from build123d import *

# Parameters (mm, degrees)
SKETCH3_W           = 20.4
SKETCH3_H           = 15.3
SKETCH3_R           = 0.5
SKETCH3_R_2         = 0.375
BOSS_EXTRUDE2_DEPTH = 0.825
SKETCH5_R           = 1
SKETCH5_R_2         = 0.5
SKETCH5_R_3         = 0.725
SKETCH5_R_4         = 0.375
BOSS_EXTRUDE3_DEPTH = 0.05


with BuildPart() as part:
    # Sketch3 → Boss-Extrude2 (new body, symmetric)
    with BuildSketch(Plane(origin=(0, 0, 0), x_dir=(1, 0, 0), z_dir=(0, 1, 0))):
        Rectangle(SKETCH3_W, SKETCH3_H)
        with Locations((-2.54, 5.11)):
            Circle(SKETCH3_R, mode=Mode.SUBTRACT)
        with Locations((0, 5.11)):
            Circle(SKETCH3_R, mode=Mode.SUBTRACT)
        with Locations((2.54, 5.11)):
            Circle(SKETCH3_R, mode=Mode.SUBTRACT)
        with Locations((-7.76, -2.57)):
            Circle(SKETCH3_R_2, mode=Mode.SUBTRACT)
        with Locations((-7.76, -5.11)):
            Circle(SKETCH3_R_2, mode=Mode.SUBTRACT)
        with Locations((7.76, -2.57)):
            Circle(SKETCH3_R_2, mode=Mode.SUBTRACT)
        with Locations((7.76, -5.11)):
            Circle(SKETCH3_R_2, mode=Mode.SUBTRACT)
        with Locations((6.260003, -3.84)):
            Circle(SKETCH3_R_2, mode=Mode.SUBTRACT)
        with Locations((-3.81, 1.3)):
            Circle(SKETCH3_R, mode=Mode.SUBTRACT)
        with Locations((3.81, 1.3)):
            Circle(SKETCH3_R, mode=Mode.SUBTRACT)
    extrude(amount=BOSS_EXTRUDE2_DEPTH, both=True)

    # Sketch5 → Boss-Extrude3 (add)
    with BuildSketch(Plane(origin=(0, 0.825, 0), x_dir=(1, 0, 0), z_dir=(0, 1, 0))):
        with Locations((-2.54, 5.11)):
            Circle(SKETCH5_R)
        with Locations((-2.54, 5.11)):
            Circle(SKETCH5_R_2, mode=Mode.SUBTRACT)
        with Locations((0, 5.11)):
            Circle(SKETCH5_R)
        with Locations((0, 5.11)):
            Circle(SKETCH5_R_2, mode=Mode.SUBTRACT)
        with Locations((2.54, 5.11)):
            Circle(SKETCH5_R)
        with Locations((2.54, 5.11)):
            Circle(SKETCH5_R_2, mode=Mode.SUBTRACT)
        with Locations((3.81, 1.3)):
            Circle(SKETCH5_R)
        with Locations((3.81, 1.3)):
            Circle(SKETCH5_R_2, mode=Mode.SUBTRACT)
        with Locations((-3.81, 1.3)):
            Circle(SKETCH5_R)
        with Locations((-3.81, 1.3)):
            Circle(SKETCH5_R_2, mode=Mode.SUBTRACT)
        with Locations((-7.76, -2.57)):
            Circle(SKETCH5_R_3)
        with Locations((-7.76, -2.57)):
            Circle(SKETCH5_R_4, mode=Mode.SUBTRACT)
        with Locations((-7.76, -5.11)):
            Circle(SKETCH5_R_3)
        with Locations((-7.76, -5.11)):
            Circle(SKETCH5_R_4, mode=Mode.SUBTRACT)
        with Locations((6.260003, -3.84)):
            Circle(SKETCH5_R_3)
        with Locations((6.260003, -3.84)):
            Circle(SKETCH5_R_4, mode=Mode.SUBTRACT)
        with Locations((7.76, -5.11)):
            Circle(SKETCH5_R_3)
        with Locations((7.76, -5.11)):
            Circle(SKETCH5_R_4, mode=Mode.SUBTRACT)
        with Locations((7.76, -2.57)):
            Circle(SKETCH5_R_3)
        with Locations((7.76, -2.57)):
            Circle(SKETCH5_R_4, mode=Mode.SUBTRACT)
    boss_extrude3 = extrude(amount=BOSS_EXTRUDE3_DEPTH)

    # Mirror1: Boss-Extrude3 across plane
    add(boss_extrude3.mirror(Plane.ZX))


solid = part.part
Geometry: final body of the model. Coordinates: model frame, mm. Give positions to 0.01 mm unless a question says otherwise; leave off trailing zeros. Loops run counter-clockwise (first coordinate to the right, second up) from the corner with the lowest first, then second, coordinate; pieces in that order, holes last. Notation, with made-up numbers: (63, -8.75) -> (117, -8.75) arc R20 ccw to (117, 16.25) -> close; hole circle Ø9 at (50.25, 7.5). An arc over 180 degrees is marked (long way). Put each result on its own line as item: value.
1. Cut plane C-C (y = -0.45). Count the separate pieces of the cut face and the enclosed holes in it, plus the area to 3 significant figures.
Taken from the geometry:
separate pieces: 1
enclosed holes: 10
area: 306 mm2
2. Pull-direction query (Z, two-part tool) for faces 1 (the flat face through (0, 0, 7.65)), 2 (the cylindrical face through (-3.04, 0.01, -5.13)), 3 (the flat face through (10.2, 0, 0)); classes: released by +Z, released by -Z, zero draft, split by the parting line, or undercut.
Taken from the geometry:
face 1: released by +Z
face 2: undercut
face 3: zero draft
3. Cut plane A-A (x = 2.54). Return the cut outline in (y, z) (3 decimals).
Taken from the geometry:
outline: (-0.875, -6.11) -> (-0.825, -6.11) -> (-0.825, -7.65) -> (0.825, -7.65) -> (0.825, -6.11) -> (0.875, -6.11) -> (0.875, -5.61) -> (-0.875, -5.61) -> close; (-0.875, -4.61) -> (0.875, -4.61) -> (0.875, -4.11) -> (0.825, -4.11) -> (0.825, 7.65) -> (-0.825, 7.65) -> (-0.825, -4.11) -> (-0.875, -4.11) -> close
4. Cut plane B-B (z = -1.3). Return the cut outline in (x, y) (3 decimals), plus the area to 3 significant figures.
Taken from the geometry:
outline: (-10.2, -0.825) -> (-4.81, -0.825) -> (-4.81, -0.875) -> (-4.31, -0.875) -> (-4.31, 0.875) -> (-4.81, 0.875) -> (-4.81, 0.825) -> (-10.2, 0.825) -> close; (-3.31, -0.875) -> (-2.81, -0.875) -> (-2.81, -0.825) -> (2.81, -0.825) -> (2.81, -0.875) -> (3.31, -0.875) -> (3.31, 0.875) -> (2.81, 0.875) -> (2.81, 0.825) -> (-2.81, 0.825) -> (-2.81, 0.875) -> (-3.31, 0.875) -> close; (4.31, -0.875) -> (4.81, -0.875) -> (4.81, -0.825) -> (10.2, -0.825) -> (10.2, 0.825) -> (4.81, 0.825) -> (4.81, 0.875) -> (4.31, 0.875) -> close
area: 30.6 mm2
5. Cut plane D-D (x = -7.76). Return the cut outline in (y, z) (3 decimals).
Taken from the geometry:
outline: (-0.875, 1.845) -> (-0.825, 1.845) -> (-0.825, -7.65) -> (0.825, -7.65) -> (0.825, 1.845) -> (0.875, 1.845) -> (0.875, 2.195) -> (-0.875, 2.195) -> close; (-0.875, 2.945) -> (0.875, 2.945) -> (0.875, 3.295) -> (0.825, 3.295) -> (0.825, 4.385) -> (0.875, 4.385) -> (0.875, 4.735) -> (-0.875, 4.735) -> (-0.875, 4.385) -> (-0.825, 4.385) -> (-0.825, 3.295) -> (-0.875, 3.295) -> close; (-0.875, 5.485) -> (0.875, 5.485) -> (0.875, 5.835) -> (0.825, 5.835) -> (0.825, 7.65) -> (-0.825, 7.65) -> (-0.825, 5.835) -> (-0.875, 5.835) -> close
6. Ray query, line 1 along Z through (x, y) = (-7.76, -0.1) (3 decimals); line 2 along X through (y, z) = (-0.4, -1.3); line 3 along Z through (x, y) = (-3.81, -0.1). Return the intervals inside material, ascending. Write a range as [from, to].
Taken from the geometry:
line 1: z = [-7.65, 2.195], [2.945, 4.735], [5.485, 7.65]
line 2: x = [-10.2, -4.31], [-3.31, 3.31], [4.31, 10.2]
line 3: z = [-7.65, -1.8], [-0.8, 7.65]
7. Pin query (flat end, axial travel): P1, Ø4.5, axis at x = -3, z = 2.5, coming from the -Y side (3 decimals); P2, Ø6, axis at x = -5.5, z = 2, coming from the -Y side (3 decimals). Return the tip coordinate at first contact, or that it passes through.
Taken from the geometry:
P1: stops at y = -0.825
P2: stops at y = -0.875
